The figure shows three views and two pictorial views of one solid part (mm, origin at its lowest corner). Answer the questions. Coordinates: 2 decimals unless noted, no trailing zeros. Order: outer loops, then holes, each group sorted by start corner. A loop starts at its lowest first (then second) coordinate and runs counter-clockwise, first axis right, second up. Notation, with made-up numbers: M 33,56 L 72,56 A28 ccw 72,93 Z; hole C 25.25,68 d7. An arc over 180 degrees is marked long. Answer in a Markdown table with one row per item. Add a question column.
Item 1: The part is cut by section B-B (y = 1.3). Write down the section's boundary in (x, z), then the cut area to 3 significant figures.
Item 2: The part is cut by section A-A (x = 2.5). Write down the section's boundary in (y, z), then the cut area to 3 significant figures.
Item 3: Consider line 1 (X direction, y = 0.8, z = 2.5); line 2 (X direction, y = 0.6, z = 23.13); line 3 (X direction, y = 0.5, z = 33.5). Determine where each line is inside the solid, lowest interval first. Write a range as from..to.
Item 4: The part is cut by section C-C (z = 34.5). Write down the section's boundary in (x, y).
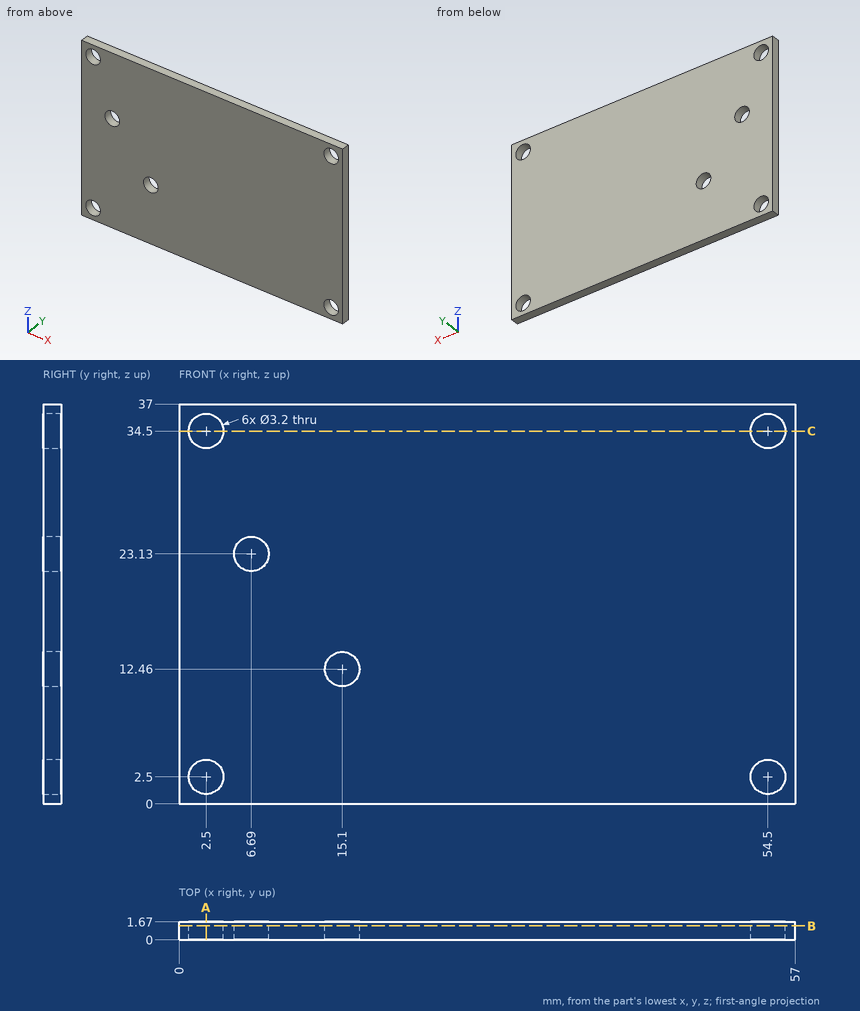
Reply:
| question | item | result |
|---|---|---|
| 1 | outline | M 0,0 L 57,0 L 57,37 L 0,37 Z; hole C 2.5,2.5 d3.2; hole C 2.5,34.5 d3.2; hole C 6.69,23.13 d3.2; hole C 15.1,12.46 d3.2; hole C 54.5,2.5 d3.2; hole C 54.5,34.5 d3.2 |
| 1 | area | 2,060 mm2 |
| 2 | outline | M 0,0 L 1.67,0 L 1.67,0.9 L 0,0.9 Z; M 0,4.1 L 1.67,4.1 L 1.67,32.9 L 0,32.9 Z; M 0,36.1 L 1.67,36.1 L 1.67,37 L 0,37 Z |
| 2 | area | 51.1 mm2 |
| 3 | line 1 | x = 0..0.9, 4.1..52.9, 56.1..57 |
| 3 | line 2 | x = 0..5.09, 8.29..57 |
| 3 | line 3 | x = 0..1.25, 3.75..53.25, 55.75..57 |
| 4 | outline | M 0,0 L 0.9,0 L 0.9,1.67 L 0,1.67 Z; M 4.1,0 L 52.9,0 L 52.9,1.67 L 4.1,1.67 Z; M 56.1,0 L 57,0 L 57,1.67 L 56.1,1.67 Z |
